Read the model definition and answer for the solid it produces. Units are mm, in the model's axes. A direction names the side the tool comes from. Coordinates: 2 decimals unless noted, no trailing zeros. Order: outer loops, then holes, each group sorted by start corner. A loop starts at its lowest first (then second) coordinate and runs counter-clockwise, first axis right, second up. Notation, with made-up numbers: M -28.75,-32 L 20.25,-32 A26 cw 20.25,1 Z; hole C 51.25,-22.5 d1. An arc over 180 degrees is marked long. Use a Markdown table: item, result. Add a question column.
1) For faces 1 (the face through (0, 61.03, 11)), 2 (the face through (-20.185, 67.075, 6.439)), 3 (the face through (0, -32, 12.7)), determine the directions among +Z, -Z, +X, -X, +Y, -Y from which every point of the face is accessible in a straight line to the end or side of a thin tool.
2) Find section C-C on z = 5.75. Count the separate pieces of the cut face and the enclosed holes in it, plus the area to 3 significant figures.
3) Find section B-B on y = 14.5. Write down the section's boundary in (x, z).
4) The mould has two halves that part along Y. Classify faces 4 (the face through (0, -19.213, 11)), 5 (the face through (0, 48, 12.7)): released by +Y, released by -Y, zero draft, split by the parting line, or undercut.
5) Each of these flat-tipped pins is pushed along its axis until it touches: pin 1 Ø0.8 at (x, y) = (3, -52.5) entering from +Z; pin 2 Ø1.4 at (x, z) = (3, 10.5) entering from -Y; pin 3 Ø4 at (y, z) = (-10.5, 11) entering from -X. Where does it stop, or does it pass through?
6) Find section A-A on x = -20.32. Write down the section's boundary in (y, z).
7) Find the intervals of material crossed by probe 1 along X at (y, z) = (23.5, 5); probe 2 along Y at (x, z) = (0, 2.5); probe 3 along Y at (x, z) = (29.5, 1), in increasing order. Write a range as [from, to].
from build123d import *

# Parameters (mm, degrees)
F0_W     = 76.2
F0_H     = 152.4
F1_DEPTH = 12.7
F2_R     = 5.08
F4_DEPTH = 25.4
F5_R     = 1.5875
F6_DEPTH = 25.4
F7_W     = 27.94
F7_H     = 1.6778
F8_DEPTH = 2.794


with BuildPart() as f1:
    # F0 (on Top) → F1 (new body)
    with BuildSketch(Plane.XY):
        Rectangle(F0_W, F0_H)
    extrude(amount=F1_DEPTH)

    # F2
    f2_edges = [f1.edges().sort_by_distance(p)[0] for p in [
        (-38.1, 0, 12.7),
        (0, 76.2, 12.7),
        (38.1, 0, 12.7),
        (0, -76.2, 12.7),
    ]]
    fillet(f2_edges, radius=F2_R)

    # F3 (on face) → F4 (cut)
    with BuildSketch(Plane.XY.offset(12.7)):
        with BuildLine():
            Line((-13.97, -61.029911), (-13.97, 61.029911))
            ThreePointArc((-13.97, 61.029911), (-20.32, 67.076798), (-26.67, 61.029911))
            Line((-26.67, 61.029911), (-26.67, -61.029911))
            ThreePointArc((-26.67, -61.029911), (-20.32, -67.076798), (-13.97, -61.029911))
        make_face()
        with BuildLine():
            ThreePointArc((26.67, 61.029911), (20.32, 67.076798), (13.97, 61.029911))
            Line((13.97, 61.029911), (13.97, -61.029911))
            ThreePointArc((13.97, -61.029911), (20.32, -67.076798), (26.67, -61.029911))
            Line((26.67, -61.029911), (26.67, 61.029911))
        make_face()
    extrude(amount=-F4_DEPTH, mode=Mode.SUBTRACT)

    # F5 (on face) → F6 (cut)
    with BuildSketch(Plane.XY.offset(12.7)):
        with Locations((0, 65.014675)):
            Circle(F5_R)
        with Locations((0, -65.014675)):
            Circle(F5_R)
        with Locations((-29.88578, 67.111924)):
            Circle(F5_R)
        with Locations((29.88578, 67.111924)):
            Circle(F5_R)
        with Locations((29.88578, -67.111924)):
            Circle(F5_R)
        with Locations((-29.88578, -67.111924)):
            Circle(F5_R)
        with Locations((-29.88578, 4.008076)):
            Circle(F5_R)
        with Locations((29.88578, 4.008076)):
            Circle(F5_R)
        with Locations((-29.88578, -4.008076)):
            Circle(F5_R)
        with Locations((29.88578, -4.008076)):
            Circle(F5_R)
    extrude(amount=-F6_DEPTH, mode=Mode.SUBTRACT)

    # F7 (on face) → F8 (cut)
    with BuildSketch(Plane.XY.offset(12.7)):
        with Locations((0, 60.191011)):
            Rectangle(F7_W, F7_H)
        with Locations((0, 52.163211)):
            Rectangle(F7_W, F7_H)
        with Locations((0, 44.135411)):
            Rectangle(F7_W, F7_H)
        with Locations((0, 36.107611)):
            Rectangle(F7_W, F7_H)
        with Locations((0, 28.079811)):
            Rectangle(F7_W, F7_H)
        with Locations((0, 20.052011)):
            Rectangle(F7_W, F7_H)
        with Locations((0, 12.024211)):
            Rectangle(F7_W, F7_H)
        with Locations((0, 3.996411)):
            Rectangle(F7_W, F7_H)
        with Locations((0, -3.996411)):
            Rectangle(F7_W, F7_H)
        with Locations((0, -12.024211)):
            Rectangle(F7_W, F7_H)
        with Locations((0, -20.052011)):
            Rectangle(F7_W, F7_H)
        with Locations((0, -28.079811)):
            Rectangle(F7_W, F7_H)
        with Locations((0, -36.107611)):
            Rectangle(F7_W, F7_H)
        with Locations((0, -44.135411)):
            Rectangle(F7_W, F7_H)
        with Locations((0, -52.163211)):
            Rectangle(F7_W, F7_H)
        with Locations((0, -60.191011)):
            Rectangle(F7_W, F7_H)
    extrude(amount=-F8_DEPTH, mode=Mode.SUBTRACT)


solid = f1.part
Check result:
| question | item | result |
|---|---|---|
| 1 | face 1 | +Z |
| 1 | face 2 | +Z, -Z |
| 1 | face 3 | +Z, +X, -X, +Y, -Y |
| 2 | separate pieces | 1 |
| 2 | enclosed holes | 12 |
| 2 | area | 8,200 mm2 |
| 3 | outline | M -38.1,0 L -26.67,0 L -26.67,12.7 L -33.02,12.7 A5.08 ccw -38.1,7.62 Z; M -13.97,0 L 13.97,0 L 13.97,12.7 L -13.97,12.7 Z; M 26.67,0 L 38.1,0 L 38.1,7.62 A5.08 ccw 33.02,12.7 L 26.67,12.7 Z |
| 4 | face 4 | undercut |
| 4 | face 5 | zero draft |
| 5 | pin 1 | stops at z = 9.91 |
| 5 | pin 2 | stops at y = -75.71 |
| 5 | pin 3 | stops at x = -37.91 |
| 6 | outline | M -76.2,0 L -67.08,0 L -67.08,12.7 L -71.12,12.7 A5.08 ccw -76.2,7.62 Z; M 67.08,0 L 76.2,0 L 76.2,7.62 A5.08 ccw 71.12,12.7 L 67.08,12.7 Z |
| 7 | probe 1 | x = [-38.1, -26.67], [-13.97, 13.97], [26.67, 38.1] |
| 7 | probe 2 | y = [-76.2, -66.6], [-63.43, 63.43], [66.6, 76.2] |
| 7 | probe 3 | y = [-76.2, -68.65], [-65.57, -5.55], [-2.47, 2.47], [5.55, 65.57], [68.65, 76.2] |
